from build123d import *

# Parameters (mm, degrees)
SKETCH1_W           = 7
SKETCH1_H           = 65.1
BOSS_EXTRUDE1_DEPTH = 2
REVOLVE1_ANGLE      = 180
SKETCH3_R           = 15
BOSS_EXTRUDE2_DEPTH = 27
SKETCH4_R           = 1.55
CUT_EXTRUDE1_DEPTH  = 2


with BuildPart() as part:
    # Sketch1 → Boss-Extrude1 (new body)
    with BuildSketch(Plane(origin=(0, 0, 0), x_dir=(1, 0, 0), z_dir=(0, 1, 0))):
        Rectangle(SKETCH1_W, SKETCH1_H)
    extrude(amount=BOSS_EXTRUDE1_DEPTH)



with BuildPart() as body_2:
    # Sketch2 → Revolve1 (revolve)
    with BuildSketch(Plane(origin=(0, 27, 0), x_dir=(1, 0, 0), z_dir=(0, 1, 0))):
        with BuildLine():
            Line((0, 15), (0, -15))
            ThreePointArc((0, -15), (15, 0), (0, 15))
        make_face()
    revolve(axis=Axis((0, 27, -15), (0, 0, 1)), revolution_arc=REVOLVE1_ANGLE)


with BuildPart() as part_1:
    add(part.part)

    add(body_2.part)  # Boss-Extrude2 merges body 2
    # Sketch3 → Boss-Extrude2 (add, through all)
    with BuildSketch(Plane.XZ.offset(-27)):
        with Locations(Location((0, 0, 0), (0, 0, 256.506601178))):
            Circle(SKETCH3_R)
    extrude(amount=BOSS_EXTRUDE2_DEPTH)

    # Sketch4 → Cut-Extrude1 (cut)
    with BuildSketch(Plane(origin=(0, 2, 0), x_dir=(1, 0, 0), z_dir=(0, 1, 0))):
        with Locations(Location((0, -28, 0), (0, 0, 270))):
            Circle(SKETCH4_R)
        with Locations(Location((0, 28, 0), (0, 0, 90))):
            Circle(SKETCH4_R)
    extrude(amount=-CUT_EXTRUDE1_DEPTH, mode=Mode.SUBTRACT)


solid = part_1.part
The model under review builds one solid part; all positions refer to its coordinate system, in mm. A direction names the side the tool comes from. Coordinates: 2 decimals unless noted, no trailing zeros. Loops run counter-clockwise (first coordinate to the right, second up) from the corner with the lowest first, then second, coordinate; pieces in that order, holes last. Notation, with made-up numbers: (-32, 16.25) -> (-7, 16.25) arc R25 ccw to (-7, 43.25) -> close; hole circle Ø10 at (50, 40). An arc over 180 degrees is marked (long way). Use a Markdown table: item, result. Add a question column.
1. Clearance check with flat-ended pins moving along their axes: pin 1 Ø3.5 at (x, z) = (0, -28) entering from +Y; pin 2 Ø10 at (x, y) = (-10.5, 5.5) entering from +Z; pin 3 Ø1.5 at (y, z) = (7.5, -11.5) entering from +X. State where each tip first meets the part, or that it passes through.
2. To check wall thickness, follow line 1 (X direction, y = 1.3, z = -28); line 2 (Y direction, x = 3, z = -29); line 3 (Z direction, x = 10.5, y = 10.5). State the ranges of each line that lie inside material, in increasing order.
3. Machinability: for faces 1 (the face through (-3.5, 1, 24)), 2 (the face through (0, 1, 32.55)), 3 (the face through (3.5, 1, 24)), 4 (the face through (0, 1, -32.55)), 5 (the face through (3.5, 1, -23)), which of the approach directions +Z, -Z, +X, -X, +Y, -Y give a long, thin tool a straight path to every point of the face, cutting with its end or side? Answer none if there is none.
4. Draft analysis for pull direction X (two halves, no side actions). For faces 6 (the face through (-0.594, 1.014, 29.432)), 7 (the face through (0, 2, 23)), 8 (the face through (-3.5, 1, -23)), state which applies: pulls with the +X half, pulls with the -X half, needs draft (parallel to the pull), parting line crosses it, or undercut.
5. Add section D-D on y = 16. Write out the cut boundary in (x, z), plus the area to 3 significant figures.
6. Add section C-C on z = -19. Write out the cut boundary in (x, y).
7. Add section B-B on z = -28. Write out the cut boundary in (x, y), plus the area to 3 significant figures.
8. Add section A-A on x = 0. Write out the cut boundary in (y, z).
Returned:
| question | item | result |
|---|---|---|
| 1 | pin 1 | stops at y = 2 |
| 1 | pin 2 | stops at z = 13.96 |
| 1 | pin 3 | stops at x = 10.46 |
| 2 | line 1 | x = -3.5 to -1.55, 1.55 to 3.5 |
| 2 | line 2 | y = 0 to 2 |
| 2 | line 3 | z = -10.71 to 10.71 |
| 3 | face 1 | +Z, -X, +Y, -Y |
| 3 | face 2 | +Z, +X, -X, +Y, -Y |
| 3 | face 3 | +Z, +X, +Y, -Y |
| 3 | face 4 | -Z, +X, -X, +Y, -Y |
| 3 | face 5 | -Z, +X, +Y, -Y |
| 4 | face 6 | undercut |
| 4 | face 7 | needs draft |
| 4 | face 8 | pulls with the -X half |
| 5 | outline | circle Ø30 at (0, 0) |
| 5 | area | 707 mm² |
| 6 | outline | (-3.5, 0) -> (3.5, 0) -> (3.5, 2) -> (-3.5, 2) -> close |
| 7 | outline | (-3.5, 0) -> (-1.55, 0) -> (-1.55, 2) -> (-3.5, 2) -> close; (1.55, 0) -> (3.5, 0) -> (3.5, 2) -> (1.55, 2) -> close |
| 7 | area | 7.80 mm² |
| 8 | outline | (0, -32.55) -> (2, -32.55) -> (2, -29.55) -> (0, -29.55) -> close; (0, -26.45) -> (2, -26.45) -> (2, -15) -> (27, -15) arc R15 ccw to (27, 15) -> (2, 15) -> (2, 26.45) -> (0, 26.45) -> close; (0, 29.55) -> (2, 29.55) -> (2, 32.55) -> (0, 32.55) -> close |
